Autodesk Inventor part; units mm, degrees
ref_plane "YZ Plane" through (0, 0, 0) normal (1, 0, 0) x (0, 1, 0)
ref_plane "XZ Plane" through (0, 0, 0) normal (0, 1, 0) x (-1, 0, 0)
ref_plane "XY Plane" through (0, 0, 0) normal (0, 0, 1) x (1, 0, 0)
sketch "Sketch1" plane through (0, 0, 0) normal (0, 0, 1) x (1, 0, 0)
  circle A0 centre (0, 0) radius 50.8 construction
  arc A1 (-100.3903, 49.8474) -> (-100.3903, -49.8474) centre (-90.5988, 0) ccw
  line L0 (-100.3903, 49.8474) -> (-44.1544, 60.8938)
  line L1 (-100.3903, -49.8474) -> (-13.1573, -66.9825)
  circle A2 centre (-74.0404, 25.4) radius 11.1125
  circle A3 centre (-74.0404, -25.4) radius 11.1125
  line L2 (-179.8386, 0) -> (89.2398, 0)
  line L3 (0, -95.9117) -> (0, 94.8458)
  line L4 (9.525, -55.1985) -> (9.525, -64.777)
  arc A4 (-13.1573, -66.9825) -> (6.6598, -67.9369) centre (0, 0) ccw
  arc A5 (-34.7181, 39.2314) -> (5.9871, -52.0443) centre (0, 0) ccw
  arc A6 (9.525, -55.1985) -> (5.9871, -52.0443) centre (6.35, -55.1985) ccw
  arc A7 (6.6598, -67.9369) -> (9.525, -64.777) centre (6.35, -64.777) ccw
  circle A8 centre (-107.95, 0) radius 14.2875
  line L5 (-107.95, -14.2875) -> (-107.95, 14.2875) construction
  line L6 (0, 0) -> (-43.7877, 43.7877) construction
  line L7 (-32.9808, 46.2166) -> (-36.9849, 56.8928)
  arc A9 (-36.9849, 56.8928) -> (-44.1544, 60.8938) centre (-42.9305, 54.6628) ccw
  arc A10 (-34.7181, 39.2314) -> (-32.9808, 46.2166) centre (-38.9264, 43.9867) ccw
  point P0 (-38.8745, 61.9309)
  point P1 (9.525, 51.5143)
  point P2 (9.525, 67.5947)
  point P3 (9.525, -51.5143)
  point P4 (9.525, -67.5947)
  point P5 (0, 52.3875)
  point P6 (-31.3803, 41.9491)
  dimension "d0" = 101.6
  dimension "d9" = 22.225
  dimension "d13" = 1.5875
  dimension "d16" = 15.875
  dimension "d28" = 50.8
  dimension "d38" = 28.575
  dimension "d39" = 107.95
  dimension "d40" = 45
  dimension "d41" = 61.9252
  dimension "d51" = 6.35
extrude "Extrusion1" add sketch "Sketch1" along normal mid plane 6.35 contours L0 A9 L7 A10 A5 L2 A8 A1 | L2 A8 A5 L3 A4 L1 A1 | L3 A5 A6 L4 A7 A4
sketch "Sketch2" plane through (0, 0, 3.175) normal (0, 0, 1) x (1, 0, 0)
  line L0 (-171.5836, 0) -> (39.7098, 0)
  line L1 (0, -94.2975) -> (0, 87.9475)
  point P0 (1.5875, 61.9125)
  point P1 (1.5875, -61.9125)
  dimension "d19" = 1.5875
  dimension "d20" = 61.9125
hole "Hole1" at (1.5875, 61.9125, 3.175) at (1.5875, -61.9125, 3.175) direction (0, 0, -1) diameter 5.1054 end through all counterbore diameter 9.779 counterbore depth 1.5875
sketch "Sketch3" plane through (0, 0, 3.175) normal (0, 0, 1) x (1, 0, 0)
  line L0 (9.525, 64.777) -> (9.525, 55.1985)
  line L1 (-100.3903, -49.8474) -> (-100.3903, 49.8474) construction
  line L2 (-171.5836, 0) -> (39.7098, 0)
  line L3 (0, -94.8704) -> (0, 91.3849)
  point P0 (-100.3903, 42.8625)
  point P1 (-100.3903, -42.8625)
  dimension "d29" = 42.8625
hole "Hole2" at (-100.3903, 42.8625, 3.175) at (-100.3903, -42.8625, 3.175) direction (0, 0, -1) diameter 5.1054 end through all counterbore diameter 9.779 counterbore depth 1.5875
sketch "Sketch4" plane through (0, 0, 3.175) normal (0, 0, 1) x (1, 0, 0)
  arc A0 (-34.7181, 39.2314) -> (5.9871, -52.0443) centre (0, 0) ccw
  line L0 (0, 0) -> (-43.7877, 43.7877) construction
  line L1 (-171.5836, 0) -> (39.7098, 0)
  line L2 (0, -94.1176) -> (0, 86.8679)
  point P0 (5.9871, 52.0443)
  dimension "d42" = 61.9252
  dimension "d43" = 45
hole "Hole3" at (-43.7877, 43.7877, 3.175) direction (0, 0, -1) diameter 5.1054 end through all counterbore diameter 9.779 counterbore depth 1.5875
properties part number "connected plate"
Geometry check sheet. Reference: the model listing, model coordinates, mm. A direction names the side the tool comes from. Round coordinates to 2 decimals unless told otherwise and drop trailing zeros. Order: outer loops, then holes, each group sorted by start corner. A loop starts at its lowest first (then second) coordinate and runs counter-clockwise, first axis right, second up. Notation, with made-up numbers: (-16, -34) -> (12, -34) arc R21 cw to (12, -24) -> close; hole circle Ø7 at (4.25, 31). An arc over 180 degrees is marked (long way). Return JSON: item names as keys, results as strings. Group by question number.
Q1. Section check A-A, the plane y = 0. Record the boundary of the cut face in (x, z) (1 decimal), plus the area to 3 significant figures.
Q2. Section check D-D, the plane x = -8. Record the boundary of the cut face in (y, z) (3 decimals), plus the area to 3 significant figures.
Q3. Release check for a two-part mould opening along Y. For faces 1 (the flat face through (-98, -45, 1.588)), 2 (the flat face through (-84, -3, -3.175)), 3 (the cylindrical face through (-32.75, 42.51, -0.04)), 4 (the cylindrical face through (-3.14, -68.19, -0.04)) record: released by +Y, released by -Y, zero draft, split by the parting line, or undercut.
Q4. Material ranges on probe 1 along X at (y, z) = (0, 1.75); probe 2 along Y at (x, z) = (-73, -0.25); probe 3 along Y at (x, z) = (-71, -0.75), recorded low to high. Write a range as from..to.
Q5. Gauge pin test, flat ends, axial feed: pin 1 (8 mm diameter, centred on x = -43.79, y = 43.79, fed in from +Z); pin 2 (4 mm diameter, centred on x = -100.39, y = -42.86, fed in from -Z) (3 decimals); pin 3 (2 mm diameter, centred on y = 25.5, z = -2, fed in from +X); pin 4 (9 mm diameter, centred on x = 1.59, y = -61.91, fed in from -Z) (3 decimals). Record the tip position at first contact, or that the pin passes through.
Q6. Section check B-B, the plane x = -107.95. Record the boundary of the cut face in (y, z) (1 decimal).
Q7. Section check C-C, the plane z = 0. Count the separate pieces of the cut face and the enclosed holes in it, plus the area to 3 significant figures.
Q8. Tool access check on faces 5 (the flat face through (-98, 41, 1.588)), 6 (the cylindrical face through (-85.142, -25.889, -0.044)). Record the directions out of +Z, -Z, +X, -X, +Y, -Y that give a thin tool (end or side, any length) a straight path to the whole face; none if there is none.
Numbers:
{
 "1": {"outline": "(-141.4, -3.2) -> (-122.2, -3.2) -> (-122.2, 3.2) -> (-141.4, 3.2) -> close; (-93.7, -3.2) -> (-52.4, -3.2) -> (-52.4, 3.2) -> (-93.7, 3.2) -> close", "area": "384 mm^2"},
 "2": {"outline": "(-67.792, -3.175) -> (-51.773, -3.175) -> (-51.773, 3.175) -> (-67.792, 3.175) -> close", "area": "102 mm^2"},
 "3": {"face 1": "undercut", "face 2": "zero draft", "face 3": "undercut", "face 4": "released by -Y"},
 "4": {"probe 1": "-141.4..-122.24, -93.66..-52.39", "probe 2": "-55.23..-36.46, -14.34..14.34, 36.46..55.23", "probe 3": "-55.62..-36.09, -14.71..14.71, 36.09..55.62"},
 "5": {"pin 1": "z = 1.59", "pin 2": "through", "pin 3": "x = -45.19", "pin 4": "z = -3.175"},
 "6": {"outline": "(-47.7, -3.2) -> (-14.3, -3.2) -> (-14.3, 3.2) -> (-47.7, 3.2) -> close; (14.3, -3.2) -> (47.7, -3.2) -> (47.7, 3.2) -> (14.3, 3.2) -> close"},
 "7": {"separate pieces": "1", "enclosed holes": "7", "area": "8,750 mm^2"},
 "8": {"face 5": "+Z", "face 6": "+Z, -Z"}
}
